Job drawing, mm, ordinate dimensions from the low corner. One solid piece. A direction names the side the tool comes from. Round coordinates to 2 decimals unless told otherwise and drop trailing zeros. Write each loop counter-clockwise with the first axis right and the second up, starting at its lowest first coordinate (ties: lowest second). Pieces come first, ordered by that corner, then holes.
1) Saw through at B-B on z = 19.5. Write the cut outline in (x, y).
2) Saw through at A-A on x = 42.5. Write the cut outline in (y, z), and give its area (3 significant figures).
3) Drill centre lines: L1, parallel to Z at x = 20.5, y = 18.5; L2, parallel to Y at x = 52, z = 10.5; L3, parallel to X at y = 4, z = 23.25. Where is each one in solid material? Low to high.
4) Saw through at D-D on y = 21. Write the cut outline in (x, z).
5) Flat gauge pins, fed straight in: pin 1 (1.5 mm diameter, centred on x = 34.5, z = 14, fed in from +Y); pin 2 (10.5 mm diameter, centred on x = 32.5, y = 18.5, fed in from -Z); pin 3 (12 mm diameter, centred on y = 16, z = 20.5, fed in from -X); pin 4 (12 mm diameter, centred on y = 13.5, z = 7.5, fed in from +X). Where does each tip first touch, or does it go through?
6) Which spindle directions (+Z, -Z, +X, -X, +Y, -Y) get a long thin tool onto all of the face, cutting with end or side? Do the marked faces 1 and 2. Say none if no direction does.
7) Saw through at C-C on x = 14.5. Write the cut outline in (y, z), and give its area (3 significant figures).
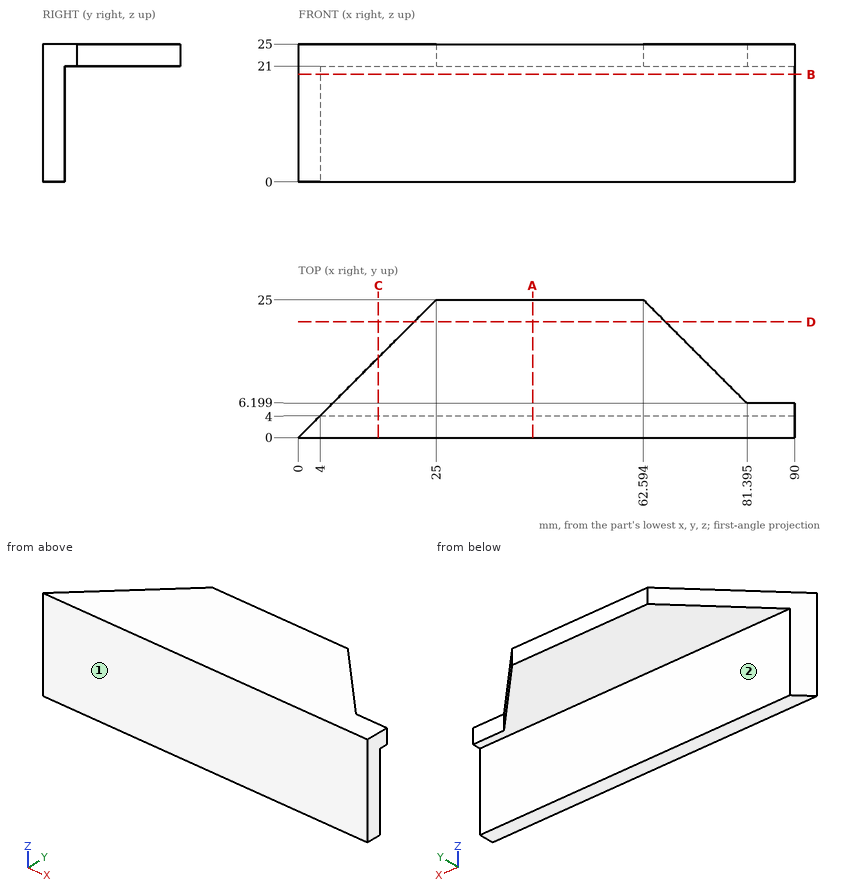
Completed:
1. outline: (0, 0) - (90, 0) - (90, 4) - (4, 4) - close
2. outline: (0, 0) - (4, 0) - (4, 21) - (25, 21) - (25, 25) - (0, 25) - close
2. area: 184 mm2
3. L1: z = 21 to 25
3. L2: y = 0 to 4
3. L3: x = 4 to 90
4. outline: (21, 21) - (66.59, 21) - (66.59, 25) - (21, 25) - close
5. pin 1: stops at y = 4
5. pin 2: stops at z = 21
5. pin 3: stops at x = 10.02
5. pin 4: passes through
6. face 1: +Z, -Z, +X, -X, -Y
6. face 2: -Z, +X, -X, +Y
7. outline: (0, 0) - (4, 0) - (4, 21) - (14.5, 21) - (14.5, 25) - (0, 25) - close
7. area: 142 mm2
